Model file for the job. Use its own axes, mm. A direction names the side the tool comes from. Coordinates: 2 decimals unless noted, no trailing zeros. Loops run counter-clockwise (first coordinate to the right, second up) from the corner with the lowest first, then second, coordinate; pieces in that order, holes last.
from build123d import *

# Parameters (mm, degrees)
SKETCH1_W           = 125.6
SKETCH1_H           = 37.2
SKETCH1_W_2         = 121.6
SKETCH1_H_2         = 33.2
BOSS_EXTRUDE1_DEPTH = 25
SKETCH2_W           = 125.6
SKETCH2_H           = 37.2
BOSS_EXTRUDE2_DEPTH = 2
SKETCH3_W           = 9
SKETCH3_H           = 9
BOSS_EXTRUDE3_DEPTH = 2
CHAMFER1_SIZE       = 9
SKETCH4_R           = 2.5
CUT_EXTRUDE1_DEPTH  = 15


with BuildPart() as part:
    # Sketch1 → Boss-Extrude1 (new body)
    with BuildSketch(Plane(origin=(0, 0, -81.397696965), x_dir=(-1, 0, 0), z_dir=(0, 0, -1))):
        with Locations((-34.603078278, 93.138059859)):
            Rectangle(SKETCH1_W, SKETCH1_H)
        with Locations((-34.603078278, 93.138059859)):
            Rectangle(SKETCH1_W_2, SKETCH1_H_2, mode=Mode.SUBTRACT)
    extrude(amount=BOSS_EXTRUDE1_DEPTH)

    # Sketch2 → Boss-Extrude2 (add)
    with BuildSketch(Plane(origin=(0, 0, -106.397696965), x_dir=(-1, 0, 0), z_dir=(0, 0, -1))):
        with Locations((-34.603078278, 93.138059859)):
            Rectangle(SKETCH2_W, SKETCH2_H)
    extrude(amount=BOSS_EXTRUDE2_DEPTH)

    # Sketch3 → Boss-Extrude3 (add)
    with BuildSketch(Plane.XY.offset(-81.397696965)):
        with Locations((90.903078278, 105.238059859)):
            Rectangle(SKETCH3_W, SKETCH3_H)
        with Locations((90.903078278, 81.038059859)):
            Rectangle(SKETCH3_W, SKETCH3_H)
        with Locations((-21.696921722, 105.238059859)):
            Rectangle(SKETCH3_W, SKETCH3_H)
        with Locations((-21.696921722, 81.038059859)):
            Rectangle(SKETCH3_W, SKETCH3_H)
    extrude(amount=-BOSS_EXTRUDE3_DEPTH)

    # Chamfer1
    chamfer1_edges = [part.edges().sort_by_distance(p)[0] for p in [
        (-21.696921722, 76.538059859, -83.397696965),
        (90.903078278, 76.538059859, -83.397696965),
        (90.903078278, 109.738059859, -83.397696965),
        (-21.696921722, 109.738059859, -83.397696965),
    ]]
    chamfer(chamfer1_edges, length=CHAMFER1_SIZE - 0.0001)  # a hair under: the kernel refuses the full size

    # Sketch4 → Cut-Extrude1 (cut)
    with BuildSketch(Plane.XY.offset(-81.397696965)):
        with Locations((-21.696921722, 105.238059859)):
            Circle(SKETCH4_R)
        with Locations((-21.696921722, 81.038059859)):
            Circle(SKETCH4_R)
        with Locations((90.903078278, 81.038059859)):
            Circle(SKETCH4_R)
        with Locations((90.903078278, 105.238059859)):
            Circle(SKETCH4_R)
    extrude(amount=-CUT_EXTRUDE1_DEPTH, mode=Mode.SUBTRACT)


solid = part.part
Q1. Flat gauge pins, fed straight in: P1, Ø3, axis at x = -21.7, y = 105.24, coming from the +Z side; P2, Ø6.5, axis at x = 90.9, y = 81.04, coming from the +Z side. Where does each tip first touch, or does it go through?
Answers:
P1: stops at z = -106.4
P2: stops at z = -81.4
Q2. Slice it at C-C (y = 89.5). List the corners of the cut face in (x, z), and give its area (3 significant figures).
Answers:
outline: (-28.2, -108.4) - (97.4, -108.4) - (97.4, -81.4) - (95.4, -81.4) - (95.4, -106.4) - (-26.2, -106.4) - (-26.2, -81.4) - (-28.2, -81.4) - close
area: 351 mm2
Q3. Slice it at A-A (z = -103.75). List the corners of the cut face in (x, y).
Answers:
outline: (-28.2, 74.54) - (97.4, 74.54) - (97.4, 111.74) - (-28.2, 111.74) - close; hole (-26.2, 76.54) - (95.4, 76.54) - (95.4, 109.74) - (-26.2, 109.74) - close
Q4. Slice it at B-B (x = 49). List the corners of the cut face in (y, z).
Answers:
outline: (74.54, -108.4) - (111.74, -108.4) - (111.74, -81.4) - (109.74, -81.4) - (109.74, -106.4) - (76.54, -106.4) - (76.54, -81.4) - (74.54, -81.4) - close
Q5. Drill centre lines: line 1 (Y direction, x = 50, z = -102.5); line 2 (X direction, y = 84, z = -86.75); line 3 (X direction, y = 78, z = -89.75). Where is each one in solid material? Low to high.
Answers:
line 1: y = 74.54 to 76.54, 109.74 to 111.74
line 2: x = -28.2 to -26.2, 95.4 to 97.4
line 3: x = -28.2 to -17.2, 86.4 to 97.4
Q6. Mould opens along Z. For faces 4 (the flat face through (-18.76, 81.101, -87.835)), 5 (the flat face through (86.403, 106, -86)), 6 (the flat face through (87.84, 105.175, -87.835)), 7 (the flat face through (35, 93, -108.398)) say: +Z half, -Z half, draft (parallel to the pull), parting line (faces both ways), or undercut.
Answers:
face 4: undercut
face 5: draft
face 6: undercut
face 7: -Z half
Q7. Which spindle directions (+Z, -Z, +X, -X, +Y, -Y) get a long thin tool onto all of the face, cutting with end or side? Do faces 1 (the flat face through (35, 109.738, -94)), 2 (the cylindrical face through (90.578, 107.717, -84.835)), 3 (the flat face through (-28.197, 93, -95)). Say none if no direction does.
Answers:
face 1: none
face 2: +Z
face 3: +Z, -Z, -X, +Y, -Y
